Work out the finished part from the listing and answer in its coordinate system (mm). A direction names the side the tool comes from. Coordinates: 2 decimals unless noted, no trailing zeros. Order: outer loops, then holes, each group sorted by start corner. A loop starts at its lowest first (then second) coordinate and runs counter-clockwise, first axis right, second up. Notation, with made-up numbers: (-24, -31.75) - (1, -31.75) arc R28 cw to (1, -10.75) - close; hole circle Ø8 at (84, 19.25). An arc over 180 degrees is marked (long way). Answer as a JSON object with one key per item and string values. Group by question number.
1) Find the intervals of material crossed by line 1 along Y through (x, z) = (-41.5, 7); line 2 along Y through (x, z) = (-40.5, 4.5); line 3 along Y through (x, z) = (-13.5, 7), in increasing order.
2) A tool of negligible diameter and unlimited length cuts with its end or side. For faces 1 (the face through (-4.977, 57, 6)), 2 (the face through (-12, 40.301, 6)), 3 (the face through (-19.8, 11.2, 6.3)), 4 (the face through (-51, 40.301, 6)), from which of +Z, -Z, +X, -X, +Y, -Y can it reach the whole face along a straight path? Write none if from no direction.
3) Section B-B (y = 27) is taken. Give the vertices of the cut face in (x, z).
4) The mould has two halves that part along Y. Classify faces 5 (the face through (-31, 45, 0)), 6 (the face through (-43.655, 11.015, 6.261)), 7 (the face through (-25.206, 39.537, 6.439)): released by +Y, released by -Y, zero draft, split by the parting line, or undercut.
5) Section C-C (z = 7.5) is taken. Give the vertices of the cut face in (x, y), plus the area to 3 significant figures.
6) Section D-D (x = -47.5) is taken. Give the vertices of the cut face in (y, z), plus the area to 3 significant figures.
7) Section A-A (x = -54) is taken. Give the vertices of the cut face in (y, z).
8) Each of these flat-tipped pins is pushed along its axis until it touches: P1, Ø5, axis at x = -15.5, z = 7.5, coming from the -Y side; P2, Ø3, axis at y = 39.5, z = 10.5, coming from the +X side; P3, Ø4, axis at y = 36, z = 6.5, coming from the -X side; P4, Ø10, axis at x = -7.5, y = 30, coming from the +Z side. Where does it stop, or does it pass through?
from build123d import *

# Parameters (mm, degrees)
F1_DEPTH = 12.7
F2_R     = 2.54
F3_R     = 2.54


with BuildPart() as f1:
    # F0 (on Top) → F1 (new body)
    with BuildSketch(Plane.XY):
        with BuildLine():
            Line((-4.977204, 46.650577), (-57.174204, 46.650577))
            Line((-57.174204, 46.650577), (-57.174204, 49.774006))
            Line((-57.174204, 49.774006), (-63.524204, 46.650577))
            Line((-63.524204, 46.650577), (-63.524204, 40.300577))
            Line((-63.524204, 40.300577), (-38.685617, 40.300577))
            Line((-38.685617, 40.300577), (-38.685617, 34.266871))
            ThreePointArc((-38.685617, 34.266871), (-48.729742, 23.719707), (-47.705534, 9.19118))
            Line((-47.705534, 9.19118), (-41.897547, 11.806156))
            ThreePointArc((-41.897547, 11.806156), (-31.839298, 29.299365), (-21.54512, 11.943945))
            Line((-21.54512, 11.943945), (-15.684392, 9.442896))
            ThreePointArc((-15.684392, 9.442896), (-15.050737, 24.39937), (-25.9308, 34.681484))
            Line((-25.9308, 34.681484), (-25.9308, 40.300577))
            Line((-25.9308, 40.300577), (1.372796, 40.300577))
            Line((1.372796, 40.300577), (1.372796, 74.057181))
            Line((1.372796, 74.057181), (-63.524204, 74.057181))
            Line((-63.524204, 74.057181), (-63.524204, 67.677669))
            Line((-63.524204, 67.677669), (-57.174204, 64.84545))
            Line((-57.174204, 64.84545), (-57.174204, 67.707181))
            Line((-57.174204, 67.707181), (-4.977204, 67.707181))
            Line((-4.977204, 67.707181), (-4.977204, 46.650577))
        make_face()
    extrude(amount=F1_DEPTH)

    # F2
    f2_edges = [f1.edges().sort_by_distance(p)[0] for p in [
        (-63.524204, 74.057181, 6.35),
        (-63.524204, 40.300577, 6.35),
        (-38.685617, 40.300577, 6.35),
        (-25.9308, 40.300577, 6.35),
        (1.372796, 40.300577, 6.35),
        (1.372796, 74.057181, 6.35),
    ]]
    fillet(f2_edges, radius=F2_R)

    # F3
    f3_edges = [f1.edges().sort_by_distance(p)[0] for p in [
        (-15.684392, 9.442896, 6.35),
        (-47.705534, 9.19118, 6.35),
    ]]
    fillet(f3_edges, radius=F3_R)


solid = f1.part
Report:
{
 "1": {"line 1": "y = 24.07 to 32.79, 40.3 to 46.65, 67.71 to 74.06", "line 2": "y = 25.37 to 33.39, 40.19 to 46.65, 67.71 to 74.06", "line 3": "y = 40.3 to 46.65, 67.71 to 74.06"},
 "2": {"face 1": "+Z, -Z", "face 2": "+Z, -Z, +X", "face 3": "+Z, -Z, -Y", "face 4": "+Z, -Z, -X"},
 "3": {"outline": "(-47.16, 0) - (-38.72, 0) - (-38.72, 12.7) - (-47.16, 12.7) - close; (-24.8, 0) - (-16.36, 0) - (-16.36, 12.7) - (-24.8, 12.7) - close"},
 "4": {"face 5": "zero draft", "face 6": "released by -Y", "face 7": "undercut"},
 "5": {"outline": "(-63.52, 42.84) arc R2.54 ccw to (-60.98, 40.3) - (-41.23, 40.3) arc R2.54 cw to (-38.69, 37.76) - (-38.69, 34.27) arc R18.03 ccw to (-48.81, 11.73) arc R2.54 ccw to (-45.36, 10.25) - (-41.9, 11.81) arc R11.68 cw (long way) to (-21.55, 11.94) - (-18.04, 10.45) arc R2.54 ccw to (-14.63, 11.99) arc R18.03 ccw to (-25.93, 34.68) - (-25.93, 37.76) arc R2.54 cw to (-23.39, 40.3) - (-1.17, 40.3) arc R2.54 ccw to (1.37, 42.84) - (1.37, 71.52) arc R2.54 ccw to (-1.17, 74.06) - (-60.98, 74.06) arc R2.54 ccw to (-63.52, 71.52) - (-63.52, 67.68) - (-57.17, 64.85) - (-57.17, 67.71) - (-4.98, 67.71) - (-4.98, 46.65) - (-57.17, 46.65) - (-57.17, 49.77) - (-63.52, 46.65) - close", "area": "1,420 mm²"},
 "6": {"outline": "(10.27, 0) - (26.42, 0) - (26.42, 12.7) - (10.27, 12.7) - close; (40.3, 0) - (46.65, 0) - (46.65, 12.7) - (40.3, 12.7) - close; (67.71, 0) - (74.06, 0) - (74.06, 12.7) - (67.71, 12.7) - close", "area": "366 mm²"},
 "7": {"outline": "(40.3, 0) - (46.65, 0) - (46.65, 12.7) - (40.3, 12.7) - close; (67.71, 0) - (74.06, 0) - (74.06, 12.7) - (67.71, 12.7) - close"},
 "8": {"P1": "stops at y = 10.24", "P2": "stops at x = 0.58", "P3": "stops at x = -39.3", "P4": "passes through"}
}
